```python
from build123d import *

# Parameters (mm, degrees)
SKETCH1_W                 = 7.5
SKETCH1_H                 = 20
SKETCH2_W                 = 1.5
SKETCH2_H                 = 10
M3X0_5_TAPPED_HOLE1_D     = 2.5
M3X0_5_TAPPED_HOLE1_DEPTH = 8.5
M3X0_5_TAPPED_HOLE1_TIP   = 0.751075774


with BuildPart() as part:
    # Sketch1 → Revolve1 (revolve)
    with BuildSketch(Plane.XY, mode=Mode.PRIVATE) as revolve1_sk:
        with Locations((16.25, 10)):
            Rectangle(SKETCH1_W, SKETCH1_H)
    revolve(revolve1_sk.sketch.rotate(Axis((0, -15.529138296, 0), (0, 1, 0)), 90), axis=Axis((0, -15.529138296, 0), (0, 1, 0)))

    # Sketch2 → Cut-Revolve1 (revolve, cut)
    with BuildSketch(Plane.XY, mode=Mode.PRIVATE) as cut_revolve1_sk:
        with Locations((13.25, 15)):
            Rectangle(SKETCH2_W, SKETCH2_H)
    revolve(cut_revolve1_sk.sketch.rotate(Axis((0, -1.547850983, 0), (0, 1, 0)), 90), axis=Axis((0, -1.547850983, 0), (0, 1, 0)), mode=Mode.SUBTRACT)

    # M3x0.5 Tapped Hole1
    with Locations(Plane(origin=(0, 20, 0), x_dir=(-1, 0, 0), z_dir=(0, 1, 0))):
        with Locations((17, 0), (-17, 0), (0, -17), (0, 17)):
            Hole(M3X0_5_TAPPED_HOLE1_D / 2, depth=M3X0_5_TAPPED_HOLE1_DEPTH)
            with Locations((0, 0, -(M3X0_5_TAPPED_HOLE1_DEPTH + M3X0_5_TAPPED_HOLE1_TIP / 2))):  # 118° drill point
                Cone(0, M3X0_5_TAPPED_HOLE1_D / 2, M3X0_5_TAPPED_HOLE1_TIP, mode=Mode.SUBTRACT)


solid = part.part
```
Work out the finished part from the listing and answer in its coordinate system (mm). A direction names the side the tool comes from. Give positions to 0.01 mm unless a question says otherwise; leave off trailing zeros. Loops run counter-clockwise (first coordinate to the right, second up) from the corner with the lowest first, then second, coordinate; pieces in that order, holes last. Notation, with made-up numbers: (64, 25) -> (105, 25) arc R19 cw to (105, 61) -> close; hole circle Ø5 at (-31, 26.25). An arc over 180 degrees is marked (long way). Put each result on its own line as item: value. Start each with the question number.
Item 1: Find the intervals of material crossed by L1, parallel to X at y = 17.75, z = 0; L2, parallel to X at y = 13.5, z = 1; L3, parallel to Y at x = 17, z = 0, in increasing order. Write a range as [from, to].
Item 2: The part is cut by section B-B (z = -12). Give the vertices of the cut face in (x, y).
Item 3: The part is cut by section A-A (y = 16). Give the vertices of the cut face in (x, z), then the cut area to 3 significant figures.
Item 4: The part is cut by section D-D (x = -13.5). Give the vertices of the cut face in (y, z).
Item 5: Each of these flat-tipped pins is pushed along its axis until it touches: P1, Ø1, axis at y = 10, z = 1, coming from the -X side; P2, Ø12, axis at x = 10, y = 11, coming from the -Z side; P3, Ø1, axis at y = 7.5, z = 14.5, coming from the +X side. Where does it stop, or does it pass through?
Item 6: Which of the six approach directions +Z, -Z, +X, -X, +Y, -Y give full straight-line access (tool end or side, diameter ignored) to faces 4 (the face through (-3.755, 5.07, -11.923)), 5 (the face through (-11.5, 10, -5.3))?
Item 7: The part is cut by section C-C (x = 4). Give the vertices of the cut face in (y, z), then the cut area to 3 significant figures.
Item 8: The mould has two halves that part along X. Classify faces 1 (the face through (-12, 20, -8)), 2 (the face through (0.672, 15.69, 18.054)), 3 (the face through (-0.88, 10.14, 19.98)): released by +X, released by -X, zero draft, split by the parting line, or undercut.
Answers below:
1. L1: [-20, -18.25], [-15.75, -14], [14, 15.75], [18.25, 20]
1. L2: [-19.97, -17.75], [-16.25, -13.96], [13.96, 16.25], [17.75, 19.97]
1. L3: [0, 10.75]
2. outline: (-16, 0) -> (-3.5, 0) -> (-3.5, 10) -> (-7.21, 10) -> (-7.21, 20) -> (-16, 20) -> close; (3.5, 0) -> (16, 0) -> (16, 20) -> (7.21, 20) -> (7.21, 10) -> (3.5, 10) -> close
3. outline: circle Ø40 at (0, 0); hole circle Ø2.5 at (-17, 0); hole circle Ø28 at (0, 0); hole circle Ø2.5 at (0, -17); hole circle Ø2.5 at (0, 17); hole circle Ø2.5 at (17, 0)
3. area: 621 mm2
4. outline: (0, -14.76) -> (20, -14.76) -> (20, -3.71) -> (10, -3.71) -> (10, 3.71) -> (20, 3.71) -> (20, 14.76) -> (0, 14.76) -> close
5. P1: x = -19.99
5. P2: z = -19.6
5. P3: x = 14.28
6. face 4: +Y, -Y
6. face 5: +Y
7. outline: (0, -19.6) -> (20, -19.6) -> (20, -13.42) -> (10, -13.42) -> (10, -11.84) -> (0, -11.84) -> close; (0, 11.84) -> (10, 11.84) -> (10, 13.42) -> (20, 13.42) -> (20, 19.6) -> (0, 19.6) -> close
7. area: 279 mm2
8. face 1: zero draft
8. face 2: undercut
8. face 3: split by the parting line
